Design review of the part shown in the three views and the two pictorial views. Dimensions are in mm from the part's minimum x, y and z. Give positions to 0.01 mm unless a question says otherwise; leave off trailing zeros. Loops run counter-clockwise (first coordinate to the right, second up) from the corner with the lowest first, then second, coordinate; pieces in that order, holes last.
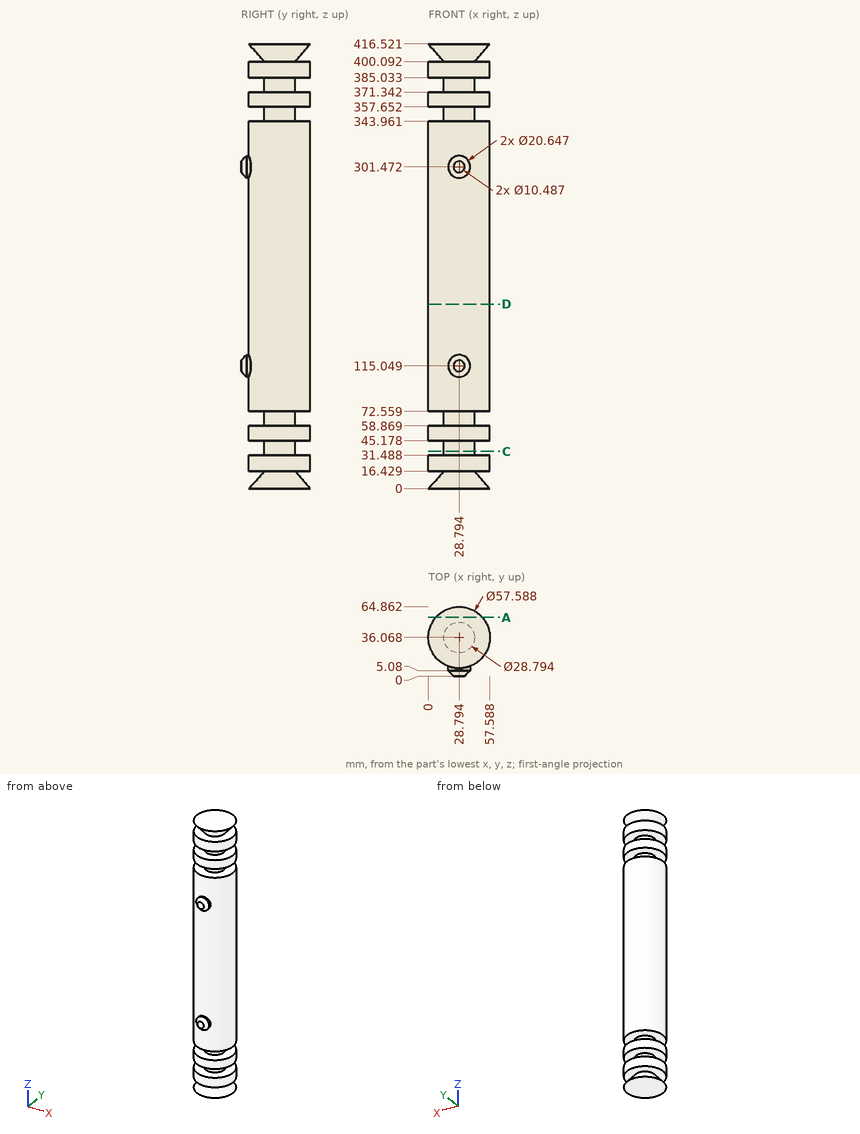
Q1. Consider section A-A on y = 55. Count the separate pieces of the cut face and the enclosed holes in it, plus the area to 3 significant figures.
Answers:
separate pieces: 7
enclosed holes: 0
area: 14,900 mm2
Q2. Consider section D-D on z = 173. Give the boundary of the cut face in (x, y) (1 decimal).
Answers:
outline: circle Ø57.6 at (28.8, 36.1)
Q3. For pin 1 Ø1.5 at (x, z) = (30, 48) entering from +Y; pin 2 Ø6 at (x, z) = (50.5, 193) entering from +Y; pin 3 Ø8 at (y, z) = (17.5, 171.5) entering from -X, all flat-tipped, find the tip position at first contact; note any pin that passes through.
Answers:
pin 1: stops at y = 64.86
pin 2: stops at y = 57.96
pin 3: stops at x = 3.96
Q4. For probe 1 along Y at (x, z) = (27, 117); probe 2 along Y at (x, z) = (45, 308.5) (1 decimal); probe 3 along X at (y, z) = (24, 98.5), list the stretches that pass through material, from the lowest coordinate up.
Answers:
probe 1: y = 0 to 64.81
probe 2: y = 12.3 to 59.9
probe 3: x = 2.65 to 54.94
Q5. Consider section C-C on z = 35. Give the boundary of the cut face in (x, y) (1 decimal), plus the area to 3 significant figures.
Answers:
outline: circle Ø28.8 at (28.8, 36.1)
area: 651 mm2
